Design review of the part shown in the three views and the two pictorial views. Dimensions are in mm from the part's minimum x, y and z. A direction names the side the tool comes from. Coordinates: 2 decimals unless noted, no trailing zeros. Write each loop counter-clockwise with the first axis right and the second up, starting at its lowest first coordinate (ties: lowest second). Pieces come first, ordered by that corner, then holes. Notation, with made-up numbers: (28, -25) - (67, -25) arc R22 ccw to (67, -2) - close; hole circle Ø2 at (63.25, 35.25). An arc over 180 degrees is marked (long way). Return JSON: item names as keys, results as strings. Group by question number.
(1) To check wall thickness, follow L1, parallel to X at y = 1, z = 1.6; L2, parallel to Y at x = 37.5, z = 2; L3, parallel to Y at x = 17.5, z = 1.35 (1 decimal). State the ranges of each line that lie inside material, in increasing order. Write a range as from..to.
(2) We need section A-A on y = 1.25. State the section outline as (x, z) points.
(3) We need section C-C on x = 14. State the section outline as (y, z) points (1 decimal).
(4) Draft analysis for pull direction X (two halves, no side actions). For the marked faces 4, 5, 6 and 7, state which applies: released by +X, released by -X, zero draft, split by the parting line, or undercut.
(5) For pin 1 Ø1.2 at (y, z) = (2, 4.5) entering from +X; pin 2 Ø6 at (x, y) = (11, 2) entering from +Z; pin 3 Ø3 at (y, z) = (6, 1) entering from +X (1 decimal); pin 4 Ø8 at (x, y) = (10, 14) entering from -Z, all flat-tipped, find the tip position at first contact; note any pin that passes through.
(6) We need section D-D on y = 5.5. State the section outline as (x, z) points.
(7) Tool access review of the marked faces 1, 2 and 3: name each direction out of +Z, -Z, +X, -X, +Y, -Y from which nothing blocks a thin tool from reaching the whole face with its end or side.
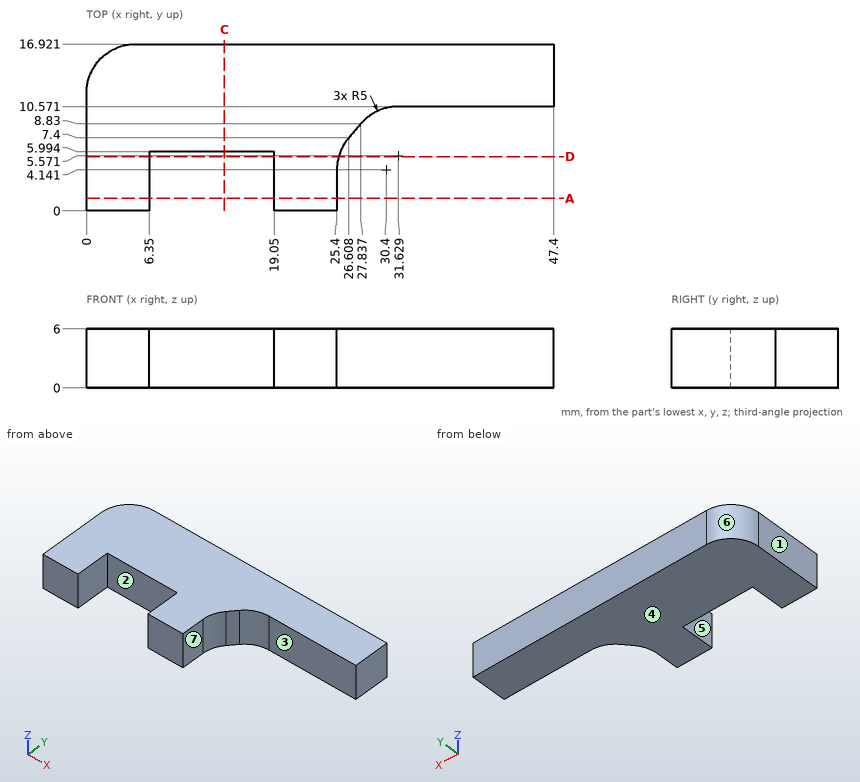
Ans:
{
 "1": {"L1": "0..6.35, 19.05..25.4", "L2": "10.57..16.92", "L3": "6..16.9"},
 "2": {"outline": "(0, 0) - (6.35, 0) - (6.35, 6) - (0, 6) - close; (19.05, 0) - (25.4, 0) - (25.4, 6) - (19.05, 6) - close"},
 "3": {"outline": "(6, 0) - (16.9, 0) - (16.9, 6) - (6, 6) - close"},
 "4": {"face 4": "zero draft", "face 5": "undercut", "face 6": "released by -X", "face 7": "released by +X"},
 "5": {"pin 1": "x = 25.4", "pin 2": "through", "pin 3": "x = 26.7", "pin 4": "z = 0"},
 "6": {"outline": "(0, 0) - (6.35, 0) - (6.35, 6) - (0, 6) - close; (19.05, 0) - (25.59, 0) - (25.59, 6) - (19.05, 6) - close"},
 "7": {"face 1": "+Z, -Z, -X, +Y, -Y", "face 2": "+Z, -Z, -Y", "face 3": "+Z, -Z, +X, -Y"}
}
